from build123d import *

# Parameters (mm, degrees)
F2_R     = 15
F2_R_2   = 10
F3_DEPTH = 12.5
F4_COUNT = 4
F4_ANGLE = 270


with BuildPart() as f1:
    # F0 (on Front) → F1 (revolve)
    with BuildSketch(Plane.XZ):
        with BuildLine():
            ThreePointArc((0, -72.5), (51.265241636, -51.265241636), (72.5, 0))
            ThreePointArc((72.5, 0), (36.024910579, 11.3389341903), (59.6428571429, -18.6809954723))
            ThreePointArc((59.6428571429, -18.6809954723), (37.0046468905, -50.3677089861), (0, -62.5))
            Line((0, -62.5), (0, -72.5))
        make_face()
    revolve(axis=Axis((0, 0, -0.3205458116), (0, 0, -1)))

    # F2 (on Front) → F3 (join, symmetric)
    with BuildSketch(Plane.XZ):
        with Locations((-72.5, 0)):
            Circle(F2_R)
        with Locations((-72.5, 0)):
            Circle(F2_R_2, mode=Mode.SUBTRACT)
    extrude(amount=F3_DEPTH, both=True)

    # F4: F1 ×4 about axis
    f4_axis = Axis((0, 0, -0.3205458116), (0, 0, 1))


with BuildPart() as f1_1:
    add(f1.part)
    for i in range(1, F4_COUNT):
        add(f1.part.rotate(f4_axis, i * F4_ANGLE / (F4_COUNT - 1)))


solid = f1_1.part
Geometry check sheet. Reference: the model listing, model coordinates, mm. Give positions to 0.01 mm unless a question says otherwise; leave off trailing zeros. Order: outer loops, then holes, each group sorted by start corner. A loop starts at its lowest first (then second) coordinate and runs counter-clockwise, first axis right, second up. Notation, with made-up numbers: M -6,28.5 L 28,28.5 A15 ccw 28,45.5 Z; hole C 31.25,28 d6. An arc over 180 degrees is marked long. Use a Markdown table: item, result.
Item 1: Section check B-B (z = -49). Record the cut outline in (x, y).
Answers follow:
| item | result |
|---|---|
| outline | C 0,0 d106.87; hole C 0,0 d77.6 |
Item 2: Section check C-C (x = -7). State how many separate pieces and enclosed holes the cut face has, and give its area (3 significant figures).
Answers follow:
| item | result |
|---|---|
| separate pieces | 1 |
| enclosed holes | 2 |
| area | 4,830 mm2 |
Item 3: Material ranges on line 1 along Y through (x, z) = (-6, 0); line 2 along Z through (x, y) = (5, 72.5); line 3 along X through (y, z) = (1.25, 0), recorded low to high.
Answers follow:
| item | result |
|---|---|
| line 1 | y = -87.5 to -82.5, -72.25 to -31.94, 31.94 to 72.25, 82.5 to 87.5 |
| line 2 | z = -15 to -10, 10 to 15 |
| line 3 | x = -87.5 to -82.5, -72.49 to -32.48, 32.48 to 72.49, 82.5 to 87.5 |
Item 4: Depth check by flat-ended pin: P1, Ø1.5, axis at y = -28, z = -9, coming from the -X side; P2, Ø17, axis at y = -81, z = -2.5, coming from the -X side; P3, Ø3, axis at x = -17.5, y = 31.5, coming from the +Z side. Enter the tip coordinate at first touch or a pass-through.
Answers follow:
| item | result |
|---|---|
| P1 | stops at x = -66.59 |
| P2 | stops at x = -12.5 |
| P3 | stops at z = 13.27 |
Item 5: Draft check along Y on faces 1 (the cylindrical face through (-0.175, -82.436, 1.133)), 2 (the flat face through (-12.5, -82.4, 2.3)), 3 (the flat face through (-82.4, 12.5, 2.3)), 4 (the flat face through (82.4, -12.5, 2.3)). Enter one of: +Y half, -Y half, draft (parallel to the pull), parting line (faces both ways), or undercut.
Answers follow:
| item | result |
|---|---|
| face 1 | undercut |
| face 2 | draft |
| face 3 | +Y half |
| face 4 | -Y half |
Item 6: Section check A-A (y = -75). Record the cut outline in (x, z), and give its area (3 significant figures).
Answers follow:
| item | result |
|---|---|
| outline | M -12.5,-14.79 L 12.5,-14.79 L 12.5,-9.68 L -12.5,-9.68 Z; M -12.5,9.68 L 12.5,9.68 L 12.5,14.79 L -12.5,14.79 Z |
| area | 255 mm2 |
